Build history of the part. All positions in model axes, mm. A direction names the side the tool comes from. Round coordinates to 2 decimals unless told otherwise and drop trailing zeros. Write each loop counter-clockwise with the first axis right and the second up, starting at its lowest first coordinate (ties: lowest second). Pieces come first, ordered by that corner, then holes.
1) Which spindle directions (+Z, -Z, +X, -X, +Y, -Y) get a long thin tool onto all of the face, cutting with end or side? Do faces 1 (the cylindrical face through (5.161, 8.095, -17.331)), 2 (the flat face through (0, 0, 18.625)), 3 (the cylindrical face through (-4.33, 3.75, 18.12)). Say none if no direction does.
2) Saw through at A-A (x = 0). Write the cut outline in (y, z) (3 decimals).
3) Saw through at C-C (x = -5). Write the cut outline in (y, z) (3 decimals).
4) Flat gauge pins, fed straight in: pin 1 (1.6 mm diameter, centred on x = 4.95, y = -4.95, fed in from +Z) (3 decimals); pin 2 (3 mm diameter, centred on x = -4.95, y = 4.95, fed in from +Z) (3 decimals); pin 3 (1 mm diameter, centred on x = 10.5, y = -7, fed in from -Z). Where does each tip first touch, or does it go through?
5) Saw through at D-D (y = -10.5). Write the cut outline in (x, z).
6) Wall check: probe 1 along Z at (x, y) = (14, 7.75); probe 2 along Y at (x, z) = (0, 17.5). Give the ranges that are in metal, low to high.
7) Saw through at B-B (y = 0). Write the cut outline in (x, z) (3 decimals), plus the area to 3 significant figures.
8) Pull direction X, two halves, no side cores. Call faces 4 (the flat face through (5, -5, 17.625)), 5 (the cylindrical face through (5.161, 8.095, 17.294)), 6 (the flat face through (17, 0, -16)): +X half, -X half, draft (parallel to the pull), parting line (faces both ways), or undercut.
from build123d import *

# Parameters (mm, degrees)
S_BOX1_W     = 45.22
S_BOX1_H     = 24.72
BOSS_1_DEPTH = 32
S_CYL2_R     = 9.6
BOSS_2_DEPTH = 3.125
S_CYL3_R     = 9.6
BOSS_3_DEPTH = 3.125
S_HOLE4_R    = 1.35
HOLE_4_DEPTH = 1.1
S_HOLE5_R    = 1.35
HOLE_5_DEPTH = 1.1
S_HOLE6_R    = 1.35
HOLE_6_DEPTH = 1.1
S_HOLE7_R    = 1.35
HOLE_7_DEPTH = 1.1


with BuildPart() as part:
    # S_box1 → Boss_1 (new body)
    with BuildSketch(Plane.XY.offset(-16)):
        with Locations((12.5, 0)):
            Rectangle(S_BOX1_W, S_BOX1_H)
    extrude(amount=BOSS_1_DEPTH)

    # S_cyl2 → Boss_2 (add)
    with BuildSketch(Plane.XY.offset(15.5)):
        Circle(S_CYL2_R)
    extrude(amount=BOSS_2_DEPTH)

    # S_cyl3 → Boss_3 (add)
    with BuildSketch(Plane.XY.offset(-18.625)):
        Circle(S_CYL3_R)
    extrude(amount=BOSS_3_DEPTH)

    # S_hole4 → Hole_4 (cut)
    with BuildSketch(Plane.XY.offset(17.625)):
        with Locations((4.949747468, 4.949747468)):
            Circle(S_HOLE4_R)
    extrude(amount=HOLE_4_DEPTH, mode=Mode.SUBTRACT)

    # S_hole5 → Hole_5 (cut)
    with BuildSketch(Plane.XY.offset(17.625)):
        with Locations((-4.949747468, 4.949747468)):
            Circle(S_HOLE5_R)
    extrude(amount=HOLE_5_DEPTH, mode=Mode.SUBTRACT)

    # S_hole6 → Hole_6 (cut)
    with BuildSketch(Plane.XY.offset(17.625)):
        with Locations((-4.949747468, -4.949747468)):
            Circle(S_HOLE6_R)
    extrude(amount=HOLE_6_DEPTH, mode=Mode.SUBTRACT)

    # S_hole7 → Hole_7 (cut)
    with BuildSketch(Plane.XY.offset(17.625)):
        with Locations((4.949747468, -4.949747468)):
            Circle(S_HOLE7_R)
    extrude(amount=HOLE_7_DEPTH, mode=Mode.SUBTRACT)


solid = part.part
Evaluation:
1. face 1: -Z
1. face 2: +Z, +X, -X, +Y, -Y
1. face 3: +Z
2. outline: (-12.36, -16) - (-9.6, -16) - (-9.6, -18.625) - (9.6, -18.625) - (9.6, -16) - (12.36, -16) - (12.36, 16) - (9.6, 16) - (9.6, 18.625) - (-9.6, 18.625) - (-9.6, 16) - (-12.36, 16) - close
3. outline: (-12.36, -16) - (-8.195, -16) - (-8.195, -18.625) - (8.195, -18.625) - (8.195, -16) - (12.36, -16) - (12.36, 16) - (8.195, 16) - (8.195, 18.625) - (6.299, 18.625) - (6.299, 17.625) - (3.601, 17.625) - (3.601, 18.625) - (-3.601, 18.625) - (-3.601, 17.625) - (-6.299, 17.625) - (-6.299, 18.625) - (-8.195, 18.625) - (-8.195, 16) - (-12.36, 16) - close
4. pin 1: stops at z = 17.625
4. pin 2: stops at z = 18.625
4. pin 3: stops at z = -16
5. outline: (-10.11, -16) - (35.11, -16) - (35.11, 16) - (-10.11, 16) - close
6. probe 1: z = -16 to 16
6. probe 2: y = -9.6 to 9.6
7. outline: (-10.11, -16) - (-9.6, -16) - (-9.6, -18.625) - (9.6, -18.625) - (9.6, -16) - (35.11, -16) - (35.11, 16) - (9.6, 16) - (9.6, 18.625) - (-9.6, 18.625) - (-9.6, 16) - (-10.11, 16) - close
7. area: 1,550 mm2
8. face 4: undercut
8. face 5: parting line
8. face 6: draft
